Geometry check sheet. Reference: the model listing, model coordinates, mm. Coordinates: 2 decimals unless noted, no trailing zeros. Order: outer loops, then holes, each group sorted by start corner. A loop starts at its lowest first (then second) coordinate and runs counter-clockwise, first axis right, second up. Notation, with made-up numbers: (36, 32.5) - (51, 32.5) arc R15 ccw to (51, 57.5) - close; hole circle Ø3 at (19.5, 66). An arc over 180 degrees is marked (long way). Use CSV: the item, a comma, the result in double quotes. Start each with the question number.
1) Sectioned sample at A-A, the plane z = -94.5. Record the cut outline in (x, y).
2) Sectioned sample at B-B, the plane x = 117. Record the cut outline in (y, z).
3) Sectioned sample at C-C, the plane x = 95.5. Record the cut outline in (y, z), and give its area (3 significant figures).
4) Depth check by flat-ended pin: P1, Ø1.5, axis at x = 122.58, z = -114.95, coming from the -Y side. Enter the tip coordinate at first touch or a pass-through.
5) Sectioned sample at D-D, the plane z = -14. Record the cut outline in (x, y), and give its area (3 significant figures).
6) Thickness scan on probe 1 along X at (y, z) = (1.1, -76.5); probe 2 along Z at (x, y) = (67, 0.55); probe 3 along Z at (x, y) = (12, 1.2). Record the ranges inside material, lowest first. Write a range as [from, to].
from build123d import *

# Parameters (mm, degrees)
SKETCH1_W                  = 134
SKETCH1_H                  = 120.35
BOSS_EXTRUDE1_DEPTH        = 2
CUT_EXTRUDE1_DEPTH         = 181.122520802
CUT_EXTRUDE2_DEPTH         = 181.122520802
LINEAR_BEARING_D           = 2.5
BELT_HOLDERS_D             = 2.5
CUT_EXTRUDE3_DEPTH         = 181.122520802
FILLET1_R                  = 5
FILLET2_R                  = 25
F_5_5_5_5_DIAMETER_HOLE1_D = 5.5


with BuildPart() as part:
    # Sketch1 → Boss-Extrude1 (new body)
    with BuildSketch(Plane(origin=(0, 0, 0), x_dir=(1, 0, 0), z_dir=(0, 1, 0))):
        with Locations((67, 60.175)):
            Rectangle(SKETCH1_W, SKETCH1_H)
    extrude(amount=BOSS_EXTRUDE1_DEPTH)

    # Sketch3 → Cut-Extrude1 (cut, through all)
    with BuildSketch(Plane(origin=(0, 2, 0), x_dir=(1, 0, 0), z_dir=(0, 1, 0))):
        with BuildLine():
            Line((86.6, 120.35), (86.6, 60))
            ThreePointArc((86.6, 60), (83.5, 56.9), (80.4, 60))
            Line((80.4, 60), (80.4, 120.35))
            Line((80.4, 120.35), (86.6, 120.35))
        make_face()
        with BuildLine():
            Line((70.1, 120.35), (70.1, 60))
            ThreePointArc((70.1, 60), (67, 56.9), (63.9, 60))
            Line((63.9, 60), (63.9, 120.35))
            Line((63.9, 120.35), (70.1, 120.35))
        make_face()
        with BuildLine():
            Line((98.6, 120.35), (98.6, 60))
            ThreePointArc((98.6, 60), (95.5, 56.9), (92.4, 60))
            Line((92.4, 60), (92.4, 120.35))
            Line((92.4, 120.35), (98.6, 120.35))
        make_face()
        with BuildLine():
            Line((58.1, 120.35), (58.1, 60))
            ThreePointArc((58.1, 60), (55, 56.9), (51.9, 60))
            Line((51.9, 60), (51.9, 120.35))
            Line((51.9, 120.35), (58.1, 120.35))
        make_face()
        with BuildLine():
            Line((41.6, 120.35), (41.6, 60))
            ThreePointArc((41.6, 60), (38.5, 56.9), (35.4, 60))
            Line((35.4, 60), (35.4, 120.35))
            Line((35.4, 120.35), (41.6, 120.35))
        make_face()
    extrude(amount=-CUT_EXTRUDE1_DEPTH, mode=Mode.SUBTRACT)

    # Sketch4 → Cut-Extrude2 (cut, through all)
    with BuildSketch(Plane(origin=(0, 2, 0), x_dir=(1, 0, 0), z_dir=(0, 1, 0))):
        with BuildLine():
            Line((47.4, 120.35), (53.6, 120.35))
            Line((53.6, 120.35), (53.6, 60))
            ThreePointArc((53.6, 60), (50.5, 56.9), (47.4, 60))
            Line((47.4, 60), (47.4, 120.35))
        make_face()
    extrude(amount=-CUT_EXTRUDE2_DEPTH, mode=Mode.SUBTRACT)

    # linear bearing (through all)
    with Locations(Plane(origin=(0, 2, 0), x_dir=(1, 0, 0), z_dir=(0, 1, 0))):
        with Locations((12, 110.35), (12, 90.35), (122, 110.35), (122, 90.35), (67, 55.35), (67, 35.35)):
            Hole(LINEAR_BEARING_D / 2)

    # belt holders (through all)
    with Locations(Plane(origin=(0, 2, 0), x_dir=(1, 0, 0), z_dir=(0, 1, 0))):
        with Locations((12, 114.95), (12, 85.75), (122.58126033, 85.75), (122.58126033, 114.95)):
            Hole(BELT_HOLDERS_D / 2)

    # Sketch9 → Cut-Extrude3 (cut, through all)
    with BuildSketch(Plane(origin=(0, 2, 0), x_dir=(1, 0, 0), z_dir=(0, 1, 0))):
        Polygon((0, 55), (50, 0), (0, 0), align=None)
        Polygon((134, 0), (134, 55), (84, 0), align=None)
    extrude(amount=-CUT_EXTRUDE3_DEPTH, mode=Mode.SUBTRACT)

    # Fillet1
    fillet1_edges = [part.edges().sort_by_distance(p)[0] for p in [
        (0, 1, -120.35),
        (134, 1, -120.35),
    ]]
    fillet(fillet1_edges, radius=FILLET1_R)

    # Fillet2
    fillet2_edges = [part.edges().sort_by_distance(p)[0] for p in [
        (0, 1, -55),
        (50, 1, 0),
        (84, 1, 0),
        (134, 1, -55),
    ]]
    fillet(fillet2_edges, radius=FILLET2_R)

    # Ø5.5 (5.5) Diameter Hole1 (through all)
    with Locations(Plane(origin=(0, 2, 0), x_dir=(1, 0, 0), z_dir=(0, 1, 0))):
        with Locations((67, 4.5), (117, 64.5), (17, 64.5)):
            Hole(F_5_5_5_5_DIAMETER_HOLE1_D / 2)


solid = part.part
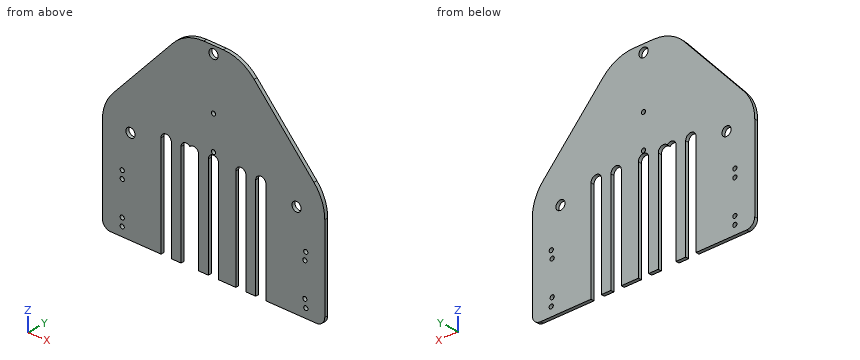
Evaluation:
1,outline,"(0, 0) - (35.4, 0) - (35.4, 2) - (0, 2) - close; (41.6, 0) - (47.4, 0) - (47.4, 2) - (41.6, 2) - close; (58.1, 0) - (63.9, 0) - (63.9, 2) - (58.1, 2) - close; (70.1, 0) - (80.4, 0) - (80.4, 2) - (70.1, 2) - close; (86.6, 0) - (92.4, 0) - (92.4, 2) - (86.6, 2) - close; (98.6, 0) - (134, 0) - (134, 2) - (98.6, 2) - close"
2,outline,"(0, -120.35) - (2, -120.35) - (2, -67.25) - (0, -67.25) - close; (0, -61.75) - (2, -61.75) - (2, -36.3) - (0, -36.3) - close"
3,outline,"(0, -56.9) - (2, -56.9) - (2, -12.65) - (0, -12.65) - close"
3,area,"88.5 mm²"
4,P1,"through"
5,outline,"(37.27, 0) - (96.73, 0) - (96.73, 2) - (37.27, 2) - close"
5,area,"119 mm²"
6,probe 1,"[0, 35.4], [41.6, 47.4], [58.1, 63.9], [70.1, 80.4], [86.6, 92.4], [98.6, 134]"
6,probe 2,"[-56.9, -56.6], [-54.1, -36.6], [-34.1, -7.25], [-1.75, 0]"
6,probe 3,"[-120.35, -116.2], [-113.7, -111.6], [-109.1, -91.6], [-89.1, -87], [-84.5, -41.8]"
